The listing builds one solid part. Answer for the finished solid, in the listing's coordinates (mm). Coordinates: 2 decimals unless noted, no trailing zeros. Loops run counter-clockwise (first coordinate to the right, second up) from the corner with the lowest first, then second, coordinate; pieces in that order, holes last. Notation, with made-up numbers: (27.25, -35) - (45.25, -35) arc R27 cw to (45.25, -13) - close; hole circle Ø8 at (-18.75, 35.5). An arc over 180 degrees is marked (long way). Write each question's results on one line, items separated by ' | '. Start each with the question number.
(1) Consider line 1 (Y direction, x = 36, z = 0.3); line 2 (Y direction, x = 50, z = 1.05); line 3 (X direction, y = -42.5, z = 0.9). Determine where each line is inside the solid, lowest interval first. Write a range as from..to.
(2) Find section D-D on z = 1.1. State how many separate pieces and enclosed holes the cut face has, then the cut area to 3 significant figures.
(3) Find section A-A on x = 44.5. Determine the outline of the cut face in (y, z), then the cut area to 3 significant figures.
(4) Find section C-C on y = -4.5. Determine the outline of the cut face in (x, z), then the cut area to 3 significant figures.
(5) Given pin 1 Ø6 at (x, y) = (103.5, -27.5) entering from +Z, flat-ended and moving along its own axis, determine where the tip first touches the part or whether it passes through.
(6) Find section B-B on y = -70.5. Determine the outline of the cut face in (x, z), then the cut area to 3 significant figures.
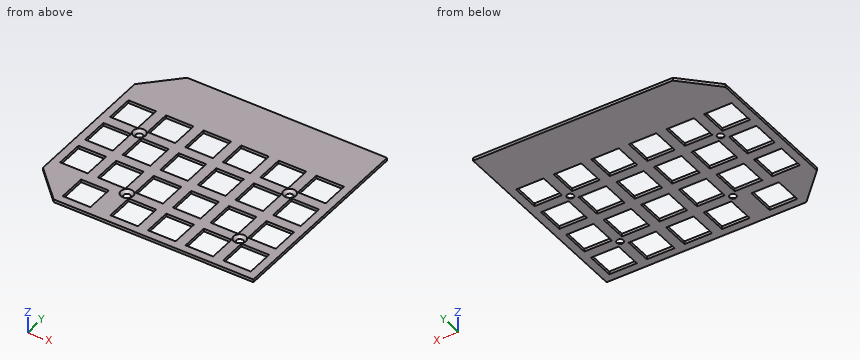
from build123d import *

# Parameters (mm, degrees)
BOSS_EXTRU_1_DEPTH                          = 1.5
ESQUISSE2_W                                 = 14
ESQUISSE2_H                                 = 14
ENL_V_MAT_EXTRU_1_DEPTH                     = 1.5
FRAISAGE_POUR_VIS_T_TE_FRAIS_E_M31_AT_COUNT = 2
FRAISAGE_POUR_VIS_T_TE_FRAIS_E_M31_AT_PITCH = 76.2
FRAISAGE_POUR_VIS_T_TE_FRAIS_E_M31_2_COUNT  = 2
FRAISAGE_POUR_VIS_T_TE_FRAIS_E_M31_2_PITCH  = 85.194189943
FRAISAGE_POUR_VIS_T_TE_FRAIS_E_M31_3_COUNT  = 2
FRAISAGE_POUR_VIS_T_TE_FRAIS_E_M31_3_PITCH  = 42.597094971


with BuildPart() as part:
    # Esquisse1 → Boss.-Extru.1 (new body)
    with BuildSketch(Plane.XY):
        Polygon((0, -85), (16, -101), (117.25, -101), (117.25, 1), (16, 1), (0, -15), align=None)
    extrude(amount=BOSS_EXTRU_1_DEPTH)

    # Esquisse2 → Enlèv. mat.-Extru.1 (cut)
    with BuildSketch(Plane.XY.offset(1.5)):
        with Locations((11, -32.85)):
            Rectangle(ESQUISSE2_W, ESQUISSE2_H)
        with Locations((30.05, -32.85)):
            Rectangle(ESQUISSE2_W, ESQUISSE2_H)
        with Locations((49.1, -32.85)):
            Rectangle(ESQUISSE2_W, ESQUISSE2_H)
        with Locations((68.15, -32.85)):
            Rectangle(ESQUISSE2_W, ESQUISSE2_H)
        with Locations((87.2, -32.85)):
            Rectangle(ESQUISSE2_W, ESQUISSE2_H)
        with Locations((106.25, -32.85)):
            Rectangle(ESQUISSE2_W, ESQUISSE2_H)
        with Locations((30.05, -51.9)):
            Rectangle(ESQUISSE2_W, ESQUISSE2_H)
        with Locations((49.1, -51.9)):
            Rectangle(ESQUISSE2_W, ESQUISSE2_H)
        with Locations((68.15, -51.9)):
            Rectangle(ESQUISSE2_W, ESQUISSE2_H)
        with Locations((87.2, -51.9)):
            Rectangle(ESQUISSE2_W, ESQUISSE2_H)
        with Locations((106.25, -51.9)):
            Rectangle(ESQUISSE2_W, ESQUISSE2_H)
        with Locations((30.05, -70.95)):
            Rectangle(ESQUISSE2_W, ESQUISSE2_H)
        with Locations((49.1, -70.95)):
            Rectangle(ESQUISSE2_W, ESQUISSE2_H)
        with Locations((68.15, -70.95)):
            Rectangle(ESQUISSE2_W, ESQUISSE2_H)
        with Locations((87.2, -70.95)):
            Rectangle(ESQUISSE2_W, ESQUISSE2_H)
        with Locations((106.25, -70.95)):
            Rectangle(ESQUISSE2_W, ESQUISSE2_H)
        with Locations((11, -51.9)):
            Rectangle(ESQUISSE2_W, ESQUISSE2_H)
        with Locations((11, -70.95)):
            Rectangle(ESQUISSE2_W, ESQUISSE2_H)
        with Locations((49.1, -90)):
            Rectangle(ESQUISSE2_W, ESQUISSE2_H)
        with Locations((68.15, -90)):
            Rectangle(ESQUISSE2_W, ESQUISSE2_H)
        with Locations((87.2, -90)):
            Rectangle(ESQUISSE2_W, ESQUISSE2_H)
        with Locations((106.25, -90)):
            Rectangle(ESQUISSE2_W, ESQUISSE2_H)
        with Locations((24.97, -90)):
            Rectangle(ESQUISSE2_W, ESQUISSE2_H)
    extrude(amount=-ENL_V_MAT_EXTRU_1_DEPTH, mode=Mode.SUBTRACT)

    # Esquisse18 → Fraisage pour vis à tête fraisée M31 (revolve, cut)
    with BuildSketch(Plane(origin=(20.525, -42.375, 1.5), x_dir=(0, -1, 0), z_dir=(1, 0, 0))):
        Polygon((0, 0), (0, 1.5), (1.7, 1.5), (1.7, 1.45), (3.15, 0), align=None)
    fraisage_pour_vis_t_te_frais_e_m31 = revolve(axis=Axis((20.525, -42.375, 7.85), (0, 0, -1)), mode=Mode.SUBTRACT)

    # Fraisage pour vis à tête fraisée M31 at: Fraisage pour vis à tête fraisée M31 ×2
    with Locations(*[(i * FRAISAGE_POUR_VIS_T_TE_FRAIS_E_M31_AT_PITCH, 0, 0) for i in range(1, FRAISAGE_POUR_VIS_T_TE_FRAIS_E_M31_AT_COUNT)]):
        add(fraisage_pour_vis_t_te_frais_e_m31, mode=Mode.SUBTRACT)

    # Fraisage pour vis _ t_te frais_e M31 2: Fraisage pour vis à tête fraisée M31 ×2
    with Locations(*[Vector(0.894427191, -0.447213595, 0) * (i * FRAISAGE_POUR_VIS_T_TE_FRAIS_E_M31_2_PITCH) for i in range(1, FRAISAGE_POUR_VIS_T_TE_FRAIS_E_M31_2_COUNT)]):
        add(fraisage_pour_vis_t_te_frais_e_m31, mode=Mode.SUBTRACT)

    # Fraisage pour vis _ t_te frais_e M31 3: Fraisage pour vis à tête fraisée M31 ×2
    with Locations(*[Vector(0.447213596, -0.894427191, 0) * (i * FRAISAGE_POUR_VIS_T_TE_FRAIS_E_M31_3_PITCH) for i in range(1, FRAISAGE_POUR_VIS_T_TE_FRAIS_E_M31_3_COUNT)]):
        add(fraisage_pour_vis_t_te_frais_e_m31, mode=Mode.SUBTRACT)


solid = part.part
Values:
1) line 1: y = -101..-77.95, -63.95..-58.9, -44.9..-39.85, -25.85..1 | line 2: y = -101..-97, -83..-77.95, -63.95..-58.9, -44.9..-39.85, -25.85..1 | line 3: x = 0..17.98, 23.07..94.18, 99.27..117.25
2) separate pieces: 1 | enclosed holes: 27 | area: 7,100 mm²
3) outline: (-101, 0) - (-97, 0) - (-97, 1.5) - (-101, 1.5) - close; (-83, 0) - (-77.95, 0) - (-77.95, 1.5) - (-83, 1.5) - close; (-63.95, 0) - (-58.9, 0) - (-58.9, 1.5) - (-63.95, 1.5) - close; (-44.9, 0) - (-39.85, 0) - (-39.85, 1.5) - (-44.9, 1.5) - close; (-25.85, 0) - (1, 0) - (1, 1.5) - (-25.85, 1.5) - close | area: 69.0 mm²
4) outline: (10.5, 0) - (117.25, 0) - (117.25, 1.5) - (10.5, 1.5) - close | area: 160 mm²
5) pin 1: stops at z = 1.5
6) outline: (0, 0) - (4, 0) - (4, 1.5) - (0, 1.5) - close; (18, 0) - (23.05, 0) - (23.05, 1.5) - (18, 1.5) - close; (37.05, 0) - (42.1, 0) - (42.1, 1.5) - (37.05, 1.5) - close; (56.1, 0) - (61.15, 0) - (61.15, 1.5) - (56.1, 1.5) - close; (75.15, 0) - (80.2, 0) - (80.2, 1.5) - (75.15, 1.5) - close; (94.2, 0) - (99.25, 0) - (99.25, 1.5) - (94.2, 1.5) - close; (113.25, 0) - (117.25, 0) - (117.25, 1.5) - (113.25, 1.5) - close | area: 49.9 mm²
